Autodesk Inventor part; units mm, degrees
ref_plane "YZ Plane" through (0, 0, 0) normal (1, 0, 0) x (0, 1, 0)
ref_plane "XZ Plane" through (0, 0, 0) normal (0, 1, 0) x (-1, 0, 0)
ref_plane "XY Plane" through (0, 0, 0) normal (0, 0, 1) x (1, 0, 0)
sketch "Sketch1" plane through (0, 0, 0) normal (0, 0, 1) x (1, 0, 0)
  circle A0 centre (0, 0) radius 5
  circle A1 centre (0, 0) radius 15
  circle A2 centre (0, 0) radius 6
  dimension "d0" = 10
  dimension "d1" = 30
  dimension "d2" = 1
extrude "Extrusion1" add sketch "Sketch1" along normal blind 1 contours A1
extrude "Extrusion2" add sketch "Sketch1" along normal blind 2 contours A2
fillet "Fillet1" radius 2 1 edges at (-6, 0, 1)
properties part number "Retenedor"
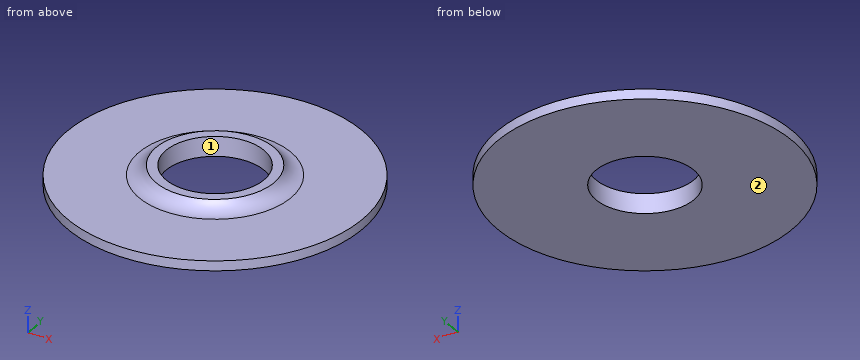
Input: part model. Units: mm. Frame: model coordinates. Face numbers are marked on the shaded views. Give positions to 0.01 mm unless a question says otherwise; leave off trailing zeros. Order: outer loops, then holes, each group sorted by start corner. A loop starts at its lowest first (then second) coordinate and runs counter-clockwise, first axis right, second up. Notation, with made-up numbers: (48.25, -34) - (88.25, -34) arc R17 cw to (88.25, -21) - close; hole circle Ø1 at (28, 72.25). An arc over 180 degrees is marked (long way). Answer as a JSON object with one key per item and string values. Group by question number.
Q1. Line query: probe 1 along Z at (x, y) = (12.75, -6.5); probe 2 along Y at (x, z) = (0.5, 1.95); probe 3 along Y at (x, z) = (0, 1.65). Output: solid intervals per line, ascending.
Q2. First-contact query: pin 1 Ø8 at (x, y) = (11, -4.5) entering from +Z; pin 2 Ø1 at (y, z) = (-5.5, 0.5) entering from +X. Flat tips, straight axial feed; report the tip coordinate or a pass-through.
Q3. Mould query, pull axis Y, two halves, no side actions, for the marked faces 1 and 2. Classes: pulls with the +Y half, pulls with the -Y half, needs draft (parallel to the pull), parting line crosses it, or undercut.
Q4. Cut plane A-A, the plane x = 0. Output: boundary loops of the cut face in (y, z).
Q5. Cut plane C-C, the plane z = 1.6. Output: boundary loops of the cut face in (x, y), then the cut area to 3 significant figures.
Q6. Cut plane D-D, the plane y = -11.5. Output: boundary loops of the cut face in (x, z), then the cut area to 3 significant figures.
Results:
{
 "1": {"probe 1": "0 to 1", "probe 2": "-6.01 to -4.97, 4.97 to 6.01", "probe 3": "-6.26 to -5, 5 to 6.26"},
 "2": {"pin 1": "z = 1", "pin 2": "x = 14.14"},
 "3": {"face 1": "undercut", "face 2": "needs draft"},
 "4": {"outline": "(-15, 0) - (-5, 0) - (-5, 2) - (-6, 2) arc R2 cw to (-7.73, 1) - (-15, 1) - close; (5, 0) - (15, 0) - (15, 1) - (7.73, 1) arc R2 cw to (6, 2) - (5, 2) - close"},
 "5": {"outline": "circle Ø12.61 at (0, 0); hole circle Ø10 at (0, 0)", "area": "46.3 mm^2"},
 "6": {"outline": "(-9.63, 0) - (9.63, 0) - (9.63, 1) - (-9.63, 1) - close", "area": "19.3 mm^2"}
}
